Here's how the part is built. I have some questions about the finished solid (model axes, mm). Round coordinates to 2 decimals unless told otherwise and drop trailing zeros. Write each loop counter-clockwise with the first axis right and the second up, starting at its lowest first coordinate (ties: lowest second). Pieces come first, ordered by that corner, then holes. Notation, with made-up numbers: (20, 17.25) -> (30, 17.25) arc R9 cw to (30, 30.25) -> close; hole circle Ø1 at (26.25, -30.5). An arc over 180 degrees is marked (long way). Answer in a Markdown table with one row per item.
from build123d import *

# Parameters (mm, degrees)
SKETCH_1_R      = 10
SKETCH_1_R_2    = 2
EXTRUDE_1_DEPTH = 2


with BuildPart() as part:
    # 草图1 → 凸台-拉伸1 (new body)
    with BuildSketch(Plane.XY):
        Polygon((317.453360513, 257.462931603), (317.453360513, 258.962931602), (314.853360513, 258.962931602), (314.853360513, 257.462931603), (311.853360513, 257.462931603), (311.853360513, 254.462931603), (314.853360513, 254.462931603), (314.853360513, 252.962931603), (317.453360513, 252.962931603), (317.453360513, 254.462931603), (319.953360513, 254.462931603), (319.953360513, 239.462931603), (321.953360513, 239.462931603), (321.953360513, 234.462931603), (319.953360513, 234.462931603), (319.953360513, 229.462931603), (321.953360513, 229.462931603), (321.953360513, 224.462931603), (319.953360513, 224.462931603), (319.953360513, 219.462931603), (319.953360513, 204.962931603), (301.453360513, 204.962931603), (301.453360513, 202.962931603), (296.453360513, 202.962931603), (296.453360513, 204.962931603), (291.453360513, 204.962931603), (291.453360513, 202.962931603), (286.453360513, 202.962931603), (286.453360513, 204.962931603), (271.453360513, 204.962931603), (271.453360513, 207.462931603), (272.953360513, 207.462931603), (272.953360513, 210.062931603), (271.453360513, 210.062931603), (271.453360513, 213.062931603), (268.453360513, 213.062931603), (268.453360513, 210.062931603), (266.953360513, 210.062931603), (266.953360513, 207.462931603), (268.453360513, 207.462931603), (268.453360513, 204.962931603), (231.453360513, 204.962931603), (231.453360513, 207.462931603), (232.953360513, 207.462931603), (232.953360513, 210.062931603), (231.453360513, 210.062931603), (231.453360513, 213.062931603), (228.453360513, 213.062931603), (228.453360513, 210.062931603), (226.953360513, 210.062931603), (226.953360513, 207.462931603), (228.453360513, 207.462931603), (228.453360513, 204.962931603), (213.453360513, 204.962931603), (213.453360513, 202.962931603), (208.453360513, 202.962931603), (208.453360513, 204.962931603), (203.453360513, 204.962931603), (203.453360513, 202.962931603), (198.453360513, 202.962931603), (198.453360513, 204.962931603), (179.953360513, 204.962931603), (179.953360513, 219.462931603), (179.953360513, 224.462931603), (177.953360513, 224.462931603), (177.953360513, 229.462931603), (179.953360513, 229.462931603), (179.953360513, 234.462931603), (177.953360513, 234.462931603), (177.953360513, 239.462931603), (179.953360513, 239.462931603), (179.953360513, 254.462931603), (182.453360513, 254.462931603), (182.453360513, 252.962931603), (185.053360513, 252.962931603), (185.053360513, 254.462931603), (188.053360513, 254.462931603), (188.053360513, 257.462931603), (185.053360513, 257.462931603), (185.053360513, 258.962931602), (182.453360513, 258.962931602), (182.453360513, 257.462931603), (179.953360513, 257.462931603), (179.953360513, 294.462931603), (182.453360513, 294.462931603), (182.453360513, 292.962931603), (185.053360513, 292.962931603), (185.053360513, 294.462931603), (188.053360513, 294.462931603), (188.053360513, 297.462931603), (185.053360513, 297.462931603), (185.053360513, 298.962931603), (182.453360513, 298.962931603), (182.453360513, 297.462931603), (179.953360513, 297.462931603), (179.953360513, 312.462931602), (177.953360513, 312.462931602), (177.953360513, 317.462931602), (179.953360513, 317.462931602), (179.953360513, 322.462931603), (177.953360513, 322.462931603), (177.953360513, 327.462931603), (179.953360513, 327.462931603), (179.953360513, 332.462931603), (179.953360513, 350.962931603), (198.453360513, 350.962931603), (198.453360513, 352.962931603), (203.453360513, 352.962931603), (203.453360513, 350.962931603), (208.453360513, 350.962931603), (208.453360513, 352.962931603), (213.453360513, 352.962931603), (213.453360513, 350.962931603), (228.453360513, 350.962931603), (228.453360513, 348.462931603), (226.953360513, 348.462931603), (226.953360513, 345.862931603), (228.453360513, 345.862931603), (228.453360513, 342.862931603), (231.453360513, 342.862931603), (231.453360513, 345.862931603), (232.953360513, 345.862931603), (232.953360513, 348.462931603), (231.453360513, 348.462931603), (231.453360513, 350.962931603), (268.453360513, 350.962931603), (268.453360513, 348.462931603), (266.953360513, 348.462931603), (266.953360513, 345.862931603), (268.453360513, 345.862931603), (268.453360513, 342.862931603), (271.453360513, 342.862931603), (271.453360513, 345.862931603), (272.953360513, 345.862931603), (272.953360513, 348.462931603), (271.453360513, 348.462931603), (271.453360513, 350.962931603), (286.453360513, 350.962931603), (286.453360513, 352.962931603), (291.453360513, 352.962931603), (291.453360513, 350.962931603), (296.453360513, 350.962931603), (296.453360513, 352.962931603), (301.453360513, 352.962931603), (301.453360513, 350.962931603), (319.953360513, 350.962931603), (319.953360513, 332.462931603), (319.953360513, 327.462931603), (321.953360513, 327.462931603), (321.953360513, 322.462931603), (319.953360513, 322.462931603), (319.953360513, 317.462931602), (321.953360513, 317.462931602), (321.953360513, 312.462931602), (319.953360513, 312.462931602), (319.953360513, 297.462931603), (317.453360513, 297.462931603), (317.453360513, 298.962931603), (314.853360513, 298.962931603), (314.853360513, 297.462931603), (311.853360513, 297.462931603), (311.853360513, 294.462931603), (314.853360513, 294.462931603), (314.853360513, 292.962931603), (317.453360513, 292.962931603), (317.453360513, 294.462931603), (319.953360513, 294.462931603), (319.953360513, 257.462931603), align=None)
        with Locations((249.953360513, 275.962931603)):
            Circle(SKETCH_1_R, mode=Mode.SUBTRACT)
        with Locations((230.953360513, 275.962931603)):
            Circle(SKETCH_1_R_2, mode=Mode.SUBTRACT)
        with Locations((236.518331671, 289.397960445)):
            Circle(SKETCH_1_R_2, mode=Mode.SUBTRACT)
        with Locations((249.953360513, 294.962931603)):
            Circle(SKETCH_1_R_2, mode=Mode.SUBTRACT)
        with Locations((263.388389356, 289.397960445)):
            Circle(SKETCH_1_R_2, mode=Mode.SUBTRACT)
        with Locations((268.953360513, 275.962931603)):
            Circle(SKETCH_1_R_2, mode=Mode.SUBTRACT)
        with Locations((263.388389356, 262.52790276)):
            Circle(SKETCH_1_R_2, mode=Mode.SUBTRACT)
        with Locations((249.953360513, 256.962931603)):
            Circle(SKETCH_1_R_2, mode=Mode.SUBTRACT)
        with Locations((236.518331671, 262.52790276)):
            Circle(SKETCH_1_R_2, mode=Mode.SUBTRACT)
        with Locations((249.953360513, 313.636994259)):
            Circle(SKETCH_1_R_2, mode=Mode.SUBTRACT)
    extrude(amount=EXTRUDE_1_DEPTH)


solid = part.part
1) I want a section at B-B, the plane y = 246. List the corners of the cut face in (x, z) for me.
Response:
| item | result |
|---|---|
| outline | (179.95, 0) -> (319.95, 0) -> (319.95, 2) -> (179.95, 2) -> close |
2) I want a section at C-C, the plane z = 0.7. Count the separate pieces of the cut face and the enclosed holes in it, and give its area (3 significant figures).
Response:
| item | result |
|---|---|
| separate pieces | 1 |
| enclosed holes | 10 |
| area | 19,900 mm^2 |
3) I want a section at D-D, the plane x = 283. List the corners of the cut face in (y, z) for me.
Response:
| item | result |
|---|---|
| outline | (204.96, 0) -> (350.96, 0) -> (350.96, 2) -> (204.96, 2) -> close |
4) I want a section at A-A, the plane x = 263.5. List the corners of the cut face in (y, z) for me.
Response:
| item | result |
|---|---|
| outline | (204.96, 0) -> (260.53, 0) -> (260.53, 2) -> (204.96, 2) -> close; (264.52, 0) -> (287.4, 0) -> (287.4, 2) -> (264.52, 2) -> close; (291.39, 0) -> (350.96, 0) -> (350.96, 2) -> (291.39, 2) -> close |
5) I need wall thicknesses on line 1 (Y direction, x = 184.5, z = 1.95); line 2 (Y direction, x = 251.5, z = 1.75); line 3 (X direction, y = 293.5, z = 0.7). Which ranges of each line are inside material? Lowest first, please. Write a range as [from, to].
Response:
| item | result |
|---|---|
| line 1 | y = [204.96, 252.96], [258.96, 292.96], [298.96, 350.96] |
| line 2 | y = [204.96, 255.69], [258.23, 266.08], [285.84, 293.69], [296.23, 312.37], [314.91, 350.96] |
| line 3 | x = [179.95, 182.45], [185.05, 248.59], [251.32, 314.85], [317.45, 319.95] |
6) We'd pull the mould along X, two halves only. Please class faces 1 (the face through (251.8, 312.87, 0.99)), 2 (the face through (251, 262, 0)): +X half, -X half, draft (parallel to the pull), parting line (faces both ways), or undercut.
Response:
| item | result |
|---|---|
| face 1 | undercut |
| face 2 | draft |
7) For pin 1 (0.8 mm diameter, centred on y = 293.5, z = 1, fed in from -X); pin 2 (1 mm diameter, centred on y = 203.5, z = 1, fed in from -X); pin 3 (0.6 mm diameter, centred on x = 178.5, z = 1.5, fed in from -Y), each with a flat end and sliding along its axis, tell me the tip position at first contact or that it passes through.
Response:
| item | result |
|---|---|
| pin 1 | stops at x = 179.95 |
| pin 2 | stops at x = 198.45 |
| pin 3 | stops at y = 224.46 |
